Work out the finished part from the listing and answer in its coordinate system (mm). Face numbers are marked on the shaded views. A direction names the side the tool comes from. Round coordinates to 2 decimals unless told otherwise and drop trailing zeros. Order: outer loops, then holes, each group sorted by start corner. A loop starts at its lowest first (then second) coordinate and runs counter-clockwise, first axis right, second up. Notation, with made-up numbers: (-28.75, 87) -> (-12.75, 87) arc R21 cw to (-12.75, 98) -> close; hole circle Ø11 at (29, 4.5). An arc over 180 degrees is marked (long way). Use one line per item in the form item = value.
```python
from build123d import *

# Parameters (mm, degrees)
CROQUIS1_R              = 1.75
SALIENTE_EXTRUIR1_DEPTH = 4
REDONDEO1_R             = 3


with BuildPart() as part:
    # Croquis1 → Saliente-Extruir1 (new body)
    with BuildSketch(Plane(origin=(0, 0, 0), x_dir=(1, 0, 0), z_dir=(0, 1, 0))):
        Polygon((0, 0), (0, 26), (6, 26), (6, 6), (34, 6), (34, 0), align=None)
        with Locations(Location((3, 23, 0), (0, 0, 270))):
            Circle(CROQUIS1_R, mode=Mode.SUBTRACT)
        with Locations(Location((31, 3, 0), (0, 0, 270))):
            Circle(CROQUIS1_R, mode=Mode.SUBTRACT)
        with Locations(Location((3, 3, 0), (0, 0, 270))):
            Circle(CROQUIS1_R, mode=Mode.SUBTRACT)
    extrude(amount=SALIENTE_EXTRUIR1_DEPTH)

    # Redondeo1
    redondeo1_edges = [part.edges().sort_by_distance(p)[0] for p in [
        (6, 2, -6),
        (0, 2, 0),
        (0, 2, -26),
        (6, 2, -26),
        (34, 2, -6),
        (34, 2, 0),
    ]]
    fillet(redondeo1_edges, radius=REDONDEO1_R - 0.0001)  # a hair under: the kernel refuses the full size


solid = part.part
```
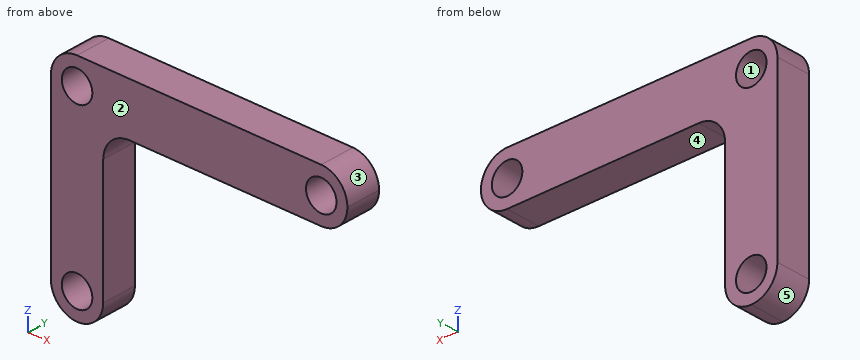
Item 1: Consider line 1 along X through (y, z) = (1.75, -3); line 2 along X through (y, z) = (2.45, -23); line 3 along X through (y, z) = (1.5, -4.5). Determine where each line is inside the solid, lowest interval first.
Findings:
line_1 = 0 to 1.25, 4.75 to 29.25, 32.75 to 34
line_2 = 0 to 1.25, 4.75 to 6
line_3 = 0 to 2.1, 3.9 to 30.1, 31.9 to 33.6
Item 2: For the marked faces 4 and 5, determine the directions among +Z, -Z, +X, -X, +Y, -Y from which every point of the face is accessible in a straight line to the end or side of a thin tool.
Findings:
face_4 = -Z, +X, +Y, -Y
face_5 = -Z, -X, +Y, -Y
Item 3: The part is cut by section B-B, the plane x = 11. Give the vertices of the cut face in (y, z), and give its area (3 significant figures).
Findings:
outline = (0, -6) -> (4, -6) -> (4, 0) -> (0, 0) -> close
area = 24.0 mm^2
Item 4: The part is cut by section A-A, the plane y = 2.35. Give the number of separate pieces and of enclosed holes in the cut face, and give its area (3 significant figures).
Findings:
separate_pieces = 1
enclosed_holes = 3
area = 287 mm^2
Item 5: The part is cut by section C-C, the plane z = -15. Give the vertices of the cut face in (x, y).
Findings:
outline = (0, 0) -> (6, 0) -> (6, 4) -> (0, 4) -> close
Item 6: A flat-ended cylindrical pin translates along its axis: P1, Ø4, axis at x = 3, z = -3, coming from the +Y side. Find the tip coordinate at first contact, or state that the pin passes through.
Findings:
P1 = 4
Item 7: Determine the mould class of the marked faces 1, 2 and 3 for opening direction Z: released by +Z, released by -Z, zero draft, split by the parting line, or undercut.
Findings:
face_1 = undercut
face_2 = zero draft
face_3 = released by +Z
